from build123d import *

# Parameters (mm, degrees)
M6_CLEARANCE_HOLE1_D     = 6.6
M6_CLEARANCE_HOLE1_DEPTH = 4
CIRPATTERN1_COUNT        = 6


with BuildPart() as part:
    # Sketch2 → Revolve1 (revolve)
    with BuildSketch(Plane.XY):
        Polygon((-7, 21), (-7, 17), (0, 17), (0, 33), (-4, 33), (-4, 21), align=None)
    revolve(axis=Axis((0, 0, 0), (-1, 0, 0)))

    # M6 Clearance Hole1
    with Locations(Plane(origin=(-4, 0, -27), x_dir=(0, -1, 0), z_dir=(-1, 0, 0))):
        with Locations((0, 0)):
            m6_clearance_hole1 = Hole(M6_CLEARANCE_HOLE1_D / 2, depth=M6_CLEARANCE_HOLE1_DEPTH)

    # CirPattern1: M6 Clearance Hole1 ×6 about axis
    cirpattern1_axis = Axis((0, 0, 0), (1, 0, 0))
    for i in range(1, CIRPATTERN1_COUNT):
        add(m6_clearance_hole1.rotate(cirpattern1_axis, i * 360 / CIRPATTERN1_COUNT), mode=Mode.SUBTRACT)


solid = part.part
Input: part model. Units: mm. Frame: model coordinates. Give positions to 0.01 mm unless a question says otherwise; leave off trailing zeros. Order: outer loops, then holes, each group sorted by start corner. A loop starts at its lowest first (then second) coordinate and runs counter-clockwise, first axis right, second up. Notation, with made-up numbers: (86.25, 36) - (128.25, 36) arc R20 cw to (128.25, 75) - close; hole circle Ø4 at (87.25, 72). An arc over 180 degrees is marked (long way). Answer as a JSON object with one key per item and string values. Group by question number.
Q1. Cut plane C-C, the plane x = -2.75. Output: boundary loops of the cut face in (y, z).
Q2. Mould query, pull axis Z, two halves, no side actions, for faces 1 (the face through (-4, 0, 22)), 2 (the face through (-5.52, 20.03, -6.31)), 3 (the face through (-1.97, -2.43, -24.77)), 4 (the face through (-1.972, -26.431, -12.236)). Classes: pulls with the +Z half, pulls with the -Z half, needs draft (parallel to the pull), parting line crosses it, or undercut.
Q3. Cut plane D-D, the plane z = -13.5. Output: boundary loops of the cut face in (x, y), then the cut area to 3 significant figures.
Q4. Line query: probe 1 along Z at (x, y) = (-1.7, 0); probe 2 along Y at (x, z) = (-3.25, -12); probe 3 along Z at (x, y) = (-3.75, 22). Output: solid intervals per line, ascending.
Q5. Cut plane A-A, the plane z = 0. Output: boundary loops of the cut face in (x, y).
Q6. Cut plane B-B, the plane y = 14. Output: boundary loops of the cut face in (x, z).
Q7. First-contact query: pin 1 Ø7.5 at (y, z) = (-23.38, 13.5) entering from -X; pin 2 Ø3 at (y, z) = (24, 25) entering from -X; pin 3 Ø2 at (y, z) = (2, -23) entering from +X; pin 4 Ø3 at (x, y) = (-1.5, -14) entering from +Z. Flat tips, straight axial feed; report the tip coordinate or a pass-through.
Results:
{
 "1": {"outline": "circle Ø66 at (0, 0); hole circle Ø6.6 at (-23.38, -13.5); hole circle Ø6.6 at (-23.38, 13.5); hole circle Ø34 at (0, 0); hole circle Ø6.6 at (0, -27); hole circle Ø6.6 at (0, 27); hole circle Ø6.6 at (23.38, -13.5); hole circle Ø6.6 at (23.38, 13.5)"},
 "2": {"face 1": "needs draft", "face 2": "parting line crosses it", "face 3": "undercut", "face 4": "undercut"},
 "3": {"outline": "(-7, -16.09) - (-4, -16.09) - (-4, -20.08) - (0, -20.08) - (0, -10.33) - (-7, -10.33) - close; (-7, 10.33) - (0, 10.33) - (0, 20.08) - (-4, 20.08) - (-4, 16.09) - (-7, 16.09) - close; (-4, -30.11) - (0, -30.11) - (0, -26.68) - (-4, -26.68) - close; (-4, 26.68) - (0, 26.68) - (0, 30.11) - (-4, 30.11) - close", "area": "140 mm^2"},
 "4": {"probe 1": "-33 to -30.3, -23.7 to -17, 17 to 23.7, 30.3 to 33", "probe 2": "-30.74 to -26.32, -20.44 to -12.04, 12.04 to 20.44, 26.32 to 30.74", "probe 3": "-24.6 to -16.5, -10.5 to 10.5, 16.5 to 24.6"},
 "5": {"outline": "(-7, -21) - (-4, -21) - (-4, -33) - (0, -33) - (0, -17) - (-7, -17) - close; (-7, 17) - (0, 17) - (0, 33) - (-4, 33) - (-4, 21) - (-7, 21) - close"},
 "6": {"outline": "(-7, -15.65) - (-4, -15.65) - (-4, -29.88) - (0, -29.88) - (0, -9.64) - (-7, -9.64) - close; (-7, 9.64) - (0, 9.64) - (0, 29.88) - (-4, 29.88) - (-4, 15.65) - (-7, 15.65) - close"},
 "7": {"pin 1": "x = -4", "pin 2": "through", "pin 3": "x = 0", "pin 4": "z = 30.54"}
}
